Answer from the drawing. Dimensions are ordinates in mm from the lowest x, y and z of the part. A direction names the side the tool comes from. Coordinates: 2 decimals unless noted, no trailing zeros. Loops run counter-clockwise (first coordinate to the right, second up) from the corner with the lowest first, then second, coordinate; pieces in that order, holes last. Notation, with made-up numbers: (-5.75, -13) -> (2.25, -13) arc R19 ccw to (2.25, 5) -> close; hole circle Ø11 at (16.25, 36). An arc over 180 degrees is marked (long way). Use a Markdown table: item, result.
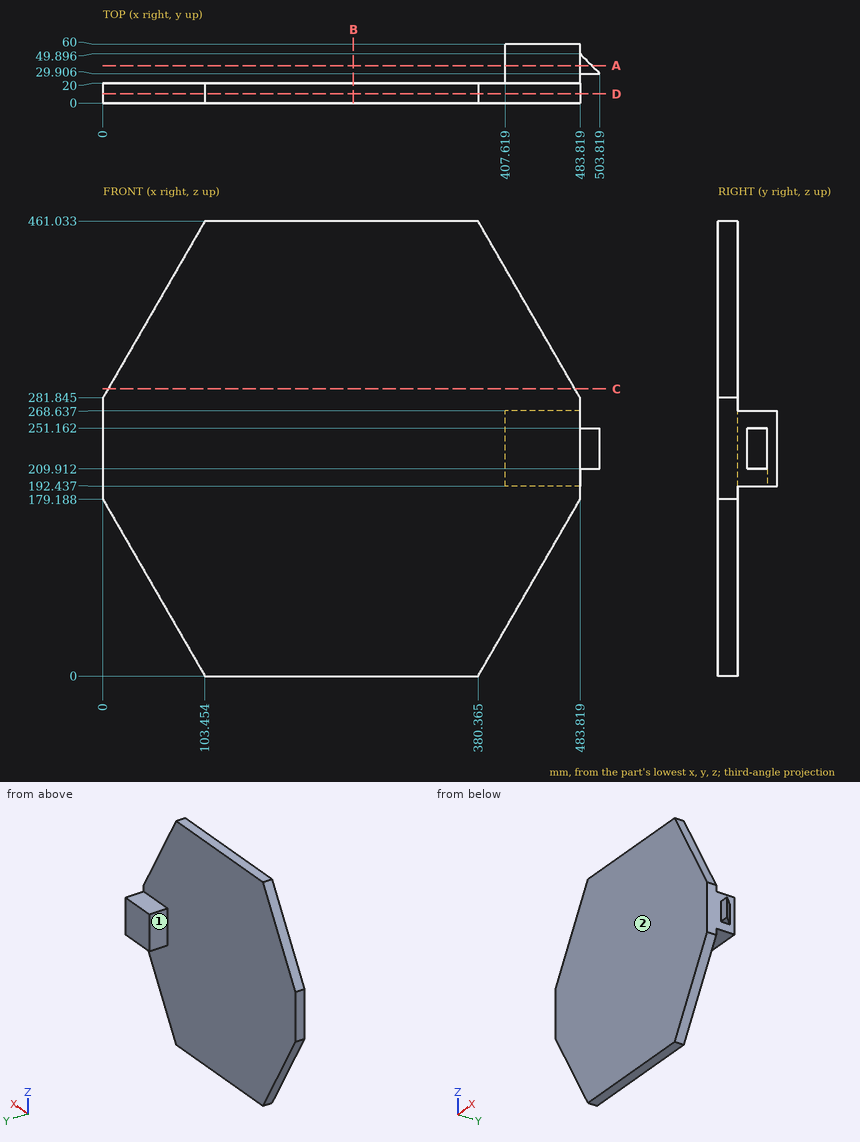
Q1. Section D-D on y = 9.5 is taken. Determine the outline of the cut face in (x, z) (1 decimal).
Solved:
| item | result |
|---|---|
| outline | (0, 179.2) -> (103.5, 0) -> (380.4, 0) -> (483.8, 179.2) -> (483.8, 281.8) -> (380.4, 461) -> (103.5, 461) -> (0, 281.8) -> close |
Q2. Given pin 1 Ø8 at (y, z) = (25, 108.5) entering from -X; pin 2 Ø3 at (y, z) = (19.5, 157) entering from -X (1 decimal); pin 3 Ø22 at (x, y) = (489.5, 41.5) entering from +Z; pin 4 Ø5 at (x, z) = (335.5, 319.5) entering from +Y, each flat-ended and moving along its own axis, determine where each tip first touches the part or whether it passes through.
Solved:
| item | result |
|---|---|
| pin 1 | through |
| pin 2 | x = 11.9 |
| pin 3 | z = 268.64 |
| pin 4 | y = 20 |
Q3. Consider line 1 (Y direction, x = 412, z = 361); line 2 (Z direction, x = 415, y = 52.5); line 3 (X direction, y = 13, z = 205.5). Determine where each line is inside the solid, lowest interval first. Write a range as [from, to].
Solved:
| item | result |
|---|---|
| line 1 | [0, 20] |
| line 2 | [192.44, 268.64] |
| line 3 | [0, 483.82] |
Q4. Section C-C on z = 291 is taken. Determine the outline of the cut face in (x, y).
Solved:
| item | result |
|---|---|
| outline | (5.29, 0) -> (478.53, 0) -> (478.53, 20) -> (5.29, 20) -> close |
Q5. Section B-B on x = 254 is taken. Determine the outline of the cut face in (y, z), and give its area (3 significant figures).
Solved:
| item | result |
|---|---|
| outline | (0, 0) -> (20, 0) -> (20, 461.03) -> (0, 461.03) -> close |
| area | 9,220 mm² |
Q6. Section A-A on y = 38 is taken. Determine the outline of the cut face in (x, z), and give its area (3 significant figures).
Solved:
| item | result |
|---|---|
| outline | (407.62, 192.44) -> (483.82, 192.44) -> (483.82, 209.91) -> (495.72, 209.91) -> (495.72, 251.16) -> (483.82, 251.16) -> (483.82, 268.64) -> (407.62, 268.64) -> close |
| area | 6,300 mm² |
Q7. For the marked faces 1 and 2, determine the directions among +Z, -Z, +X, -X, +Y, -Y from which every point of the face is accessible in a straight line to the end or side of a thin tool.
Solved:
| item | result |
|---|---|
| face 1 | +Z, -Z, -X, +Y |
| face 2 | +Z, -Z, +X, -X, -Y |
